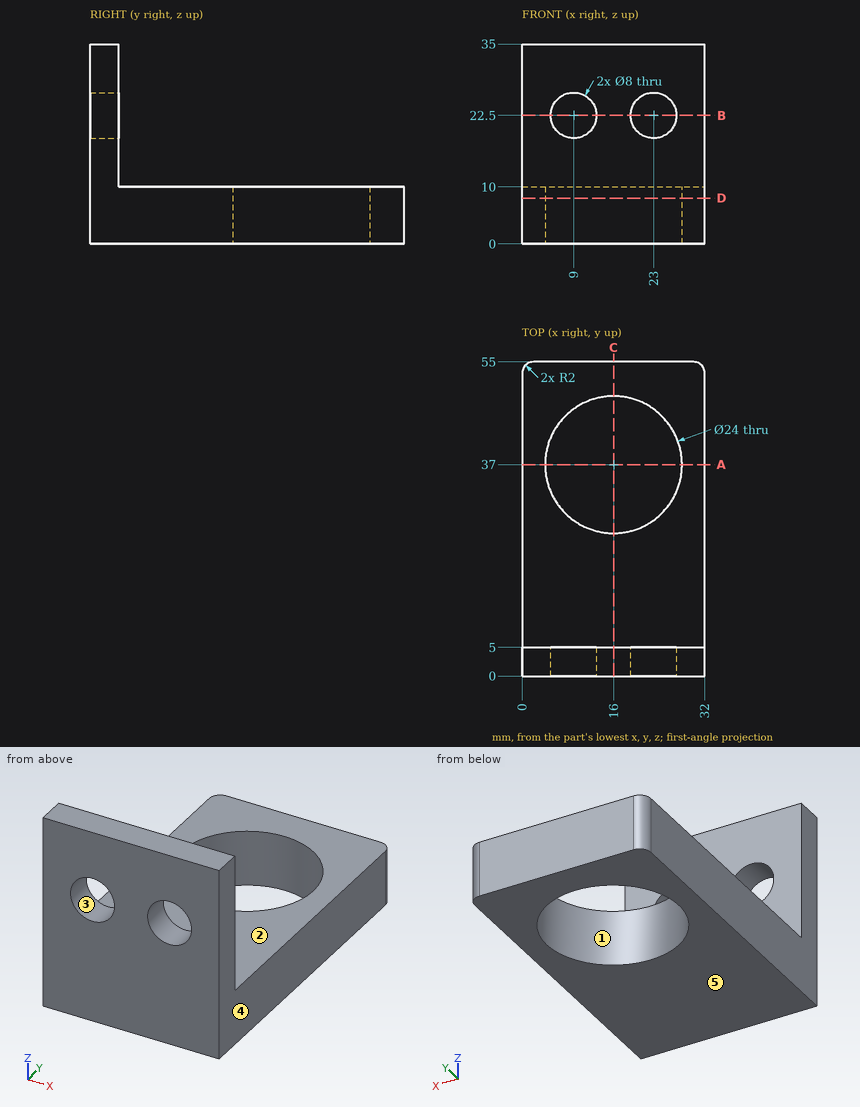
Design review of the part shown in the three views and the two pictorial views. Dimensions are in mm from the part's minimum x, y and z. A direction names the side the tool comes from. Coordinates: 2 decimals unless noted, no trailing zeros. Loops run counter-clockwise (first coordinate to the right, second up) from the corner with the lowest first, then second, coordinate; pieces in that order, holes last.
Q1. We need section A-A on y = 37. State the section outline as (x, z) points.
Reported:
outline: (0, 0) - (4, 0) - (4, 10) - (0, 10) - close; (28, 0) - (32, 0) - (32, 10) - (28, 10) - close
Q2. We need section D-D on z = 8. State the section outline as (x, y) points, and give its area (3 significant figures).
Reported:
outline: (0, 0) - (32, 0) - (32, 53) arc R2 ccw to (30, 55) - (2, 55) arc R2 ccw to (0, 53) - close; hole circle Ø24 at (16, 37)
area: 1,310 mm2
Q3. We need section B-B on z = 22.5. State the section outline as (x, y) points, and give its area (3 significant figures).
Reported:
outline: (0, 0) - (5, 0) - (5, 5) - (0, 5) - close; (13, 0) - (19, 0) - (19, 5) - (13, 5) - close; (27, 0) - (32, 0) - (32, 5) - (27, 5) - close
area: 80.0 mm2
Q4. We need section C-C on x = 16. State the section outline as (y, z) points.
Reported:
outline: (0, 0) - (25, 0) - (25, 10) - (5, 10) - (5, 35) - (0, 35) - close; (49, 0) - (55, 0) - (55, 10) - (49, 10) - close
Q5. For pin 1 (10 mm diameter, centred on y = 33.5, z = 17.5, fed in from -X); pin 2 (10.5 mm diameter, centred on x = 23, z = 22.5, fed in from +Y); pin 3 (6 mm diameter, centred on x = 26.5, y = 11, fed in from +Z), all flat-tipped, find the tip position at first contact; note any pin that passes through.
Reported:
pin 1: passes through
pin 2: stops at y = 5
pin 3: stops at z = 10
Q6. Tool access review of the marked faces 1 and 2: name each direction out of +Z, -Z, +X, -X, +Y, -Y from which nothing blocks a thin tool from reaching the whole face with its end or side.
Reported:
face 1: +Z, -Z
face 2: +Z, +X, -X, +Y
Q7. To check wall thickness, follow line 1 (Z direction, x = 9, y = 2.1); line 2 (X direction, y = 2.25, z = 22.5); line 3 (Y direction, x = 16, z = 6.5). State the ranges of each line that lie inside material, in increasing order.
Reported:
line 1: z = 0 to 18.5, 26.5 to 35
line 2: x = 0 to 5, 13 to 19, 27 to 32
line 3: y = 0 to 25, 49 to 55
Q8. The part is to be moulded in two halves that separate along X. For the marked faces 3, 4 and 5, say which applies: +X half, -X half, draft (parallel to the pull), parting line (faces both ways), or undercut.
Reported:
face 3: undercut
face 4: +X half
face 5: draft
